Geometry: final body of the model. Coordinates: model frame, mm. A direction names the side the tool comes from. Give positions to 0.01 mm unless a question says otherwise; leave off trailing zeros. Write each loop counter-clockwise with the first axis right and the second up, starting at its lowest first coordinate (ties: lowest second). Pieces come first, ordered by that corner, then holes. Notation, with made-up numbers: M 86,12.25 L 134,12.25 A14 cw 134,36.25 Z; hole C 63.25,85 d7. An arc over 180 degrees is marked long. Use a Markdown table: item, result. Add a question column.
(1) Cut plane D-D (x = -8.25). Output: boundary loops of the cut face in (y, z), plus the area to 3 significant figures.
(2) Draft query along X for faces 4 (the flat face through (10.5, -1, 4)), 5 (the cylindrical face through (-0.26, -5.028, -12.517)), 6 (the flat face through (0, 17, 10)). Return one class per face: released by +X, released by -X, zero draft, split by the parting line, or undercut.
(3) Cut plane C-C (y = -1). Output: boundary loops of the cut face in (x, z).
(4) Cut plane A-A (z = 9). Output: boundary loops of the cut face in (x, y).
(5) Pin query (flat end, axial travel): pin 1 Ø5.5 at (x, y) = (8.5, 11) entering from -Z; pin 2 Ø4 at (x, z) = (4.5, -1.5) entering from +Y; pin 3 Ø2.5 at (x, z) = (-0.5, -13.5) entering from +Y. Return the tip coordinate at first contact, or that it passes through.
(6) Reachability of faces 1 (the cylindrical face through (0, -5, 16.5)), 2 (the flat face through (0, 0, -5)), 3 (the cylindrical face through (0.87, 16.01, 10.59)) from +Z, -Z, +X, -X, +Y, -Y: full face, straight path, thin tool, end or side. Return the list, or none.
(7) Material intervals for L1, parallel to Z at x = 0, y = -5.6; L2, parallel to Z at x = 0, y = -1.4; L3, parallel to Z at x = 0, y = 15.9, sorted ascending.
(8) Cut plane B-B (x = 0). State how many separate pieces and enclosed holes the cut face has, plus the area to 3 significant figures.
```python
from build123d import *

# Parameters (mm, degrees)
F0_W      = 21
F0_H      = 42
F1_DEPTH  = 7
F2_W      = 21
F2_H      = 5
F3_DEPTH  = 17
F4_R      = 2
F5_DEPTH  = 25
F6_R      = 4
F7_DEPTH  = 3
F8_R      = 4
F9_DEPTH  = 25
F10_W     = 21
F10_H     = 2
F11_DEPTH = 15
F12_R     = 2
F13_DEPTH = 25
F14_R     = 4
F15_DEPTH = 5


with BuildPart() as f1:
    # F0 (on Front) → F1 (new body)
    with BuildSketch(Plane.XZ):
        Rectangle(F0_W, F0_H)
    extrude(amount=F1_DEPTH)

    # F2 (on face) → F3 (join)
    with BuildSketch(Plane(origin=(0, 0, 0), x_dir=(-1, 0, 0), z_dir=(0, 1, 0))):
        with Locations((0, 18.5)):
            Rectangle(F2_W, F2_H)
    extrude(amount=F3_DEPTH)

    # F4 (on face) → F5 (cut)
    with BuildSketch(Plane.XZ.offset(7)):
        with Locations((0, 14.5)):
            Circle(F4_R)
        with Locations((0, -14.5)):
            Circle(F4_R)
    extrude(amount=-F5_DEPTH, mode=Mode.SUBTRACT)

    # F6 (on face) → F7 (cut)
    with BuildSketch(Plane(origin=(0, 0, 0), x_dir=(-1, 0, 0), z_dir=(0, 1, 0))):
        with Locations((0, 14.520681)):
            Circle(F6_R)
        with Locations((0, -14.510261)):
            Circle(F6_R)
    extrude(amount=-F7_DEPTH, mode=Mode.SUBTRACT)

    # F8 (on face) → F9 (cut)
    with BuildSketch(Plane.XZ):
        with Locations((0, 14.548728)):
            Circle(F8_R)
    extrude(amount=-F9_DEPTH, mode=Mode.SUBTRACT)

    # F10 (on face) → F11 (join)
    with BuildSketch(Plane.XY.offset(21)):
        with Locations((0, 16)):
            Rectangle(F10_W, F10_H)
    extrude(amount=-F11_DEPTH)

    # F12 (on face) → F13 (cut)
    with BuildSketch(Plane.XZ.offset(7)):
        with Locations((0, 14.492556)):
            Circle(F12_R)
    extrude(amount=-F13_DEPTH, mode=Mode.SUBTRACT)

    # F14 (on face) → F15 (cut)
    with BuildSketch(Plane(origin=(0, 17, 0), x_dir=(-1, 0, 0), z_dir=(0, 1, 0))):
        with Locations((0, 14.492556)):
            Circle(F14_R)
    extrude(amount=-F15_DEPTH, mode=Mode.SUBTRACT)


solid = f1.part
```
Answer list:
| question | item | result |
|---|---|---|
| 1 | outline | M -7,-21 L 0,-21 L 0,16 L 15,16 L 15,6 L 17,6 L 17,21 L -7,21 Z |
| 1 | area | 399 mm² |
| 2 | face 4 | released by +X |
| 2 | face 5 | undercut |
| 2 | face 6 | zero draft |
| 3 | outline | M -10.5,-21 L 10.5,-21 L 10.5,21 L -10.5,21 Z; hole C 0,-14.51 d8; hole C 0,14.52 d8 |
| 4 | outline | M -10.5,-7 L 10.5,-7 L 10.5,0 L -10.5,0 Z; M -10.5,15 L 10.5,15 L 10.5,17 L -10.5,17 Z |
| 5 | pin 1 | z = 16 |
| 5 | pin 2 | y = 0 |
| 5 | pin 3 | y = -3 |
| 6 | face 1 | +Y, -Y |
| 6 | face 2 | -Z, +X, -X |
| 6 | face 3 | +Y |
| 7 | L1 | -21 to -16.5, -12.5 to 12.49, 16.5 to 21 |
| 7 | L2 | -21 to -18.51, -10.51 to 10.52, 18.52 to 21 |
| 7 | L3 | 6 to 10.49, 18.49 to 21 |
| 8 | separate pieces | 4 |
| 8 | enclosed holes | 0 |
| 8 | area | 265 mm² |
